from build123d import *

# Parameters (mm, degrees)
SKETCH2_W           = 78.8
SKETCH2_H           = 244.1
SKETCH2_W_2         = 55
SKETCH2_H_2         = 3.5
BOSS_EXTRUDE1_DEPTH = 2
SKETCH3_W           = 2
SKETCH3_H           = 244.1
BOSS_EXTRUDE2_DEPTH = 50
FILLET1_R           = 1.5
SKETCH4_W           = 16
SKETCH4_H           = 40.5
CUT_EXTRUDE1_DEPTH  = 27507.713596192


with BuildPart() as part:
    # Sketch2 → Boss-Extrude1 (new body)
    with BuildSketch(Plane(origin=(0, 27504.249263039, 0), x_dir=(1, 0, 0), z_dir=(0, 1, 0))):
        with Locations((-7.2, 17)):
            Rectangle(SKETCH2_W, SKETCH2_H)
        with Locations((-7.2, 123.528571429)):
            Rectangle(SKETCH2_W_2, SKETCH2_H_2, mode=Mode.SUBTRACT)
        with Locations((-7.2, 134.65)):
            Rectangle(SKETCH2_W_2, SKETCH2_H_2, mode=Mode.SUBTRACT)
        with Locations((-7.2, 112.407142857)):
            Rectangle(SKETCH2_W_2, SKETCH2_H_2, mode=Mode.SUBTRACT)
        with Locations((-7.2, 101.285714286)):
            Rectangle(SKETCH2_W_2, SKETCH2_H_2, mode=Mode.SUBTRACT)
        with Locations((-7.2, 90.164285714)):
            Rectangle(SKETCH2_W_2, SKETCH2_H_2, mode=Mode.SUBTRACT)
        with Locations((-7.2, 79.042857143)):
            Rectangle(SKETCH2_W_2, SKETCH2_H_2, mode=Mode.SUBTRACT)
        with Locations((-7.2, 67.921428571)):
            Rectangle(SKETCH2_W_2, SKETCH2_H_2, mode=Mode.SUBTRACT)
        with Locations((-7.2, 56.8)):
            Rectangle(SKETCH2_W_2, SKETCH2_H_2, mode=Mode.SUBTRACT)
        with Locations((-7.2, 45.678571429)):
            Rectangle(SKETCH2_W_2, SKETCH2_H_2, mode=Mode.SUBTRACT)
        with Locations((-7.2, 34.557142857)):
            Rectangle(SKETCH2_W_2, SKETCH2_H_2, mode=Mode.SUBTRACT)
        with Locations((-7.2, 23.435714286)):
            Rectangle(SKETCH2_W_2, SKETCH2_H_2, mode=Mode.SUBTRACT)
        with Locations((-7.2, 12.314285714)):
            Rectangle(SKETCH2_W_2, SKETCH2_H_2, mode=Mode.SUBTRACT)
        with Locations((-7.2, 1.192857143)):
            Rectangle(SKETCH2_W_2, SKETCH2_H_2, mode=Mode.SUBTRACT)
        with Locations((-7.2, -9.928571429)):
            Rectangle(SKETCH2_W_2, SKETCH2_H_2, mode=Mode.SUBTRACT)
        with Locations((-7.2, -21.05)):
            Rectangle(SKETCH2_W_2, SKETCH2_H_2, mode=Mode.SUBTRACT)
        with Locations((-7.2, -32.171428571)):
            Rectangle(SKETCH2_W_2, SKETCH2_H_2, mode=Mode.SUBTRACT)
        with Locations((-7.2, -43.292857143)):
            Rectangle(SKETCH2_W_2, SKETCH2_H_2, mode=Mode.SUBTRACT)
        with Locations((-7.2, -54.414285714)):
            Rectangle(SKETCH2_W_2, SKETCH2_H_2, mode=Mode.SUBTRACT)
        with Locations((-7.2, -65.535714286)):
            Rectangle(SKETCH2_W_2, SKETCH2_H_2, mode=Mode.SUBTRACT)
        with Locations((-7.2, -76.657142857)):
            Rectangle(SKETCH2_W_2, SKETCH2_H_2, mode=Mode.SUBTRACT)
        with Locations((-7.2, -87.778571429)):
            Rectangle(SKETCH2_W_2, SKETCH2_H_2, mode=Mode.SUBTRACT)
        with Locations((-7.2, -98.9)):
            Rectangle(SKETCH2_W_2, SKETCH2_H_2, mode=Mode.SUBTRACT)
    extrude(amount=BOSS_EXTRUDE1_DEPTH)

    # Sketch3 → Boss-Extrude2 (add)
    with BuildSketch(Plane.XZ.offset(-27504.249263039)):
        with Locations((-45.6, -17)):
            Rectangle(SKETCH3_W, SKETCH3_H)
        with Locations((31.2, -17)):
            Rectangle(SKETCH3_W, SKETCH3_H)
    extrude(amount=BOSS_EXTRUDE2_DEPTH)

    # Fillet1
    fillet1_edges = [part.edges().sort_by_distance(p)[0] for p in [
        (32.2, 27506.249263039, -17),
        (-44.6, 27504.249263039, -17),
        (30.2, 27504.249263039, -17),
        (-46.6, 27506.249263039, -17),
    ]]
    fillet(fillet1_edges, radius=FILLET1_R)

    # Sketch4 → Cut-Extrude1 (cut, through all)
    with BuildSketch(Plane(origin=(32.2, 0, 0), x_dir=(0, 0, -1), z_dir=(1, 0, 0))):
        with Locations((-89.05, 27480.499263039)):
            Rectangle(SKETCH4_W, SKETCH4_H)
        with Locations((-65.483333333, 27480.499263039)):
            Rectangle(SKETCH4_W, SKETCH4_H)
        with Locations((-41.916666667, 27480.499263039)):
            Rectangle(SKETCH4_W, SKETCH4_H)
        with Locations((-18.35, 27480.499263039)):
            Rectangle(SKETCH4_W, SKETCH4_H)
        with Locations((5.216666667, 27480.499263039)):
            Rectangle(SKETCH4_W, SKETCH4_H)
        with Locations((28.783333333, 27480.499263039)):
            Rectangle(SKETCH4_W, SKETCH4_H)
        with Locations((52.35, 27480.499263039)):
            Rectangle(SKETCH4_W, SKETCH4_H)
        with Locations((75.916666667, 27480.499263039)):
            Rectangle(SKETCH4_W, SKETCH4_H)
        with Locations((99.483333333, 27480.499263039)):
            Rectangle(SKETCH4_W, SKETCH4_H)
        with Locations((123.05, 27480.499263039)):
            Rectangle(SKETCH4_W, SKETCH4_H)
    extrude(amount=-CUT_EXTRUDE1_DEPTH, mode=Mode.SUBTRACT)


solid = part.part
Work out the finished part from the listing and answer in its coordinate system (mm). A direction names the side the tool comes from. Give positions to 0.01 mm unless a question says otherwise; leave off trailing zeros. One line per item, written item: value.
Item 1: Find section A-A, the plane y = 27473.5. State how many separate pieces and enclosed holes the cut face has, plus the area to 3 significant figures.
Answer sheet:
separate pieces: 22
enclosed holes: 0
area: 336 mm²
Item 2: Flat-ended cylindrical pins translate along their axes: P1, Ø0.6, axis at y = 27505.5, z = -90.5, coming from the -X side; P2, Ø10, axis at x = 13, z = -37, coming from the -Y side. Find the tip coordinate at first contact, or state that the pin passes through.
Answer sheet:
P1: x = -46.53
P2: y = 27504.25
Item 3: A tool of negligible diameter and unlimited length cuts with its end or side. For faces 1 (the flat face through (-8, 27504.249, -19)), 2 (the flat face through (32.2, 27479, -15)), from which of +Z, -Z, +X, -X, +Y, -Y can it reach the whole face along a straight path? Write none if from no direction.
Answer sheet:
face 1: +Z, -Z, -Y
face 2: +Z, -Z, +X, +Y, -Y
Item 4: Straight lines are drawn through the part: probe 1 along X at (y, z) = (27480.5, -115); probe 2 along Y at (x, z) = (-28, -37). For each, find the intervals that lie inside material, in ascending order.
Answer sheet:
probe 1: -46.6 to -44.6, 30.2 to 32.2
probe 2: 27504.25 to 27506.25
Item 5: Determine the mould class of faces 3 (the flat face through (-46.6, 27480, -19)), 4 (the flat face through (30.2, 27475, -18)), 5 (the flat face through (-7, 27505, -139.05)) for opening direction X: released by +X, released by -X, zero draft, split by the parting line, or undercut.
Answer sheet:
face 3: released by -X
face 4: undercut
face 5: zero draft
